Can you work these out from the model? Positions are in its coordinate system, mm. Face numbers are marked on the shaded views. A direction names the side the tool comes from. Round coordinates to 2 decimals unless told otherwise and drop trailing zeros. Order: outer loops, then holes, each group sorted by start corner. A loop starts at its lowest first (then second) coordinate and runs counter-clockwise, first axis right, second up. Notation, with made-up numbers: (89, -10) -> (143, -10) arc R18 cw to (143, 25) -> close; hole circle Ø2 at (58.25, 33). An arc over 180 degrees is marked (long way). One line per item, written item: value.
```python
from build123d import *

# Parameters (mm, degrees)
F0_W     = 40
F0_H     = 40
F1_DEPTH = 40
F2_W     = 20
F2_H     = 20
F3_DEPTH = 20
F7_DEPTH = 24.4958974278


with BuildPart() as f1:
    # F0 (on Front) → F1 (new body)
    with BuildSketch(Plane.XZ):
        with Locations((20, 20)):
            Rectangle(F0_W, F0_H)
    extrude(amount=F1_DEPTH)

    # F2 (on face) → F3 (cut)
    with BuildSketch(Plane.XZ.offset(40)):
        with Locations((30, 30)):
            Rectangle(F2_W, F2_H)
    extrude(amount=-F3_DEPTH, mode=Mode.SUBTRACT)

    # F6 (on 3pt) → F7 (cut, through all)
    with BuildSketch(Plane(origin=(16.6666666667, -16.6666666667, 33.3333333333), x_dir=(0.9128709292, 0.1825741858, -0.3651483717), z_dir=(-0.4082482905, 0.4082482905, -0.8164965809))):
        Polygon((3.6514837167, 26.83281573), (25.5603860169, 8.94427191), (25.5603860169, 31.304951685), align=None)
    extrude(amount=-F7_DEPTH, mode=Mode.SUBTRACT)


solid = f1.part
```
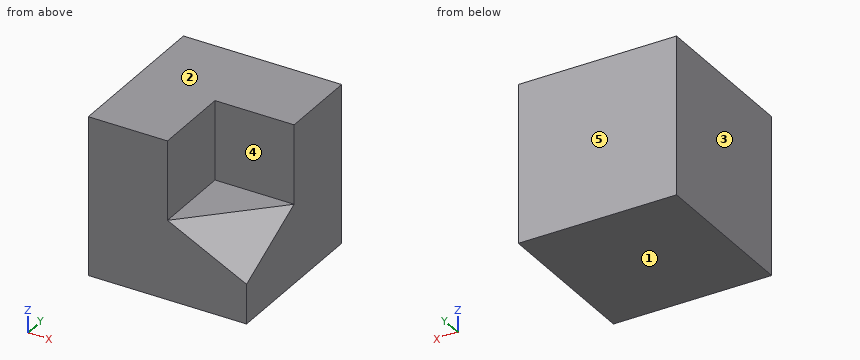
Q1. I want a section at B-B on x = 27. List the corners of the cut face in (y, z) for me.
Answers below:
outline: (-40, 0) -> (0, 0) -> (0, 40) -> (-20, 40) -> (-20, 20) -> (-33, 20) -> (-40, 16.5) -> close
Q2. Will these pins go through, and if not, where does the flat tip stop? pin 1 Ø12 at (y, z) = (-35, 20.5) entering from +X; pin 2 Ø16 at (y, z) = (-31.5, 33.5) entering from +X; pin 3 Ø6 at (x, y) = (27, -26) entering from +Z.
Answers below:
pin 1: x = 37.42
pin 2: x = 20
pin 3: z = 20
Q3. I want a section at D-D on z = 14. List the corners of the cut face in (x, y) for me, plus the area to 3 significant figures.
Answers below:
outline: (0, -40) -> (32, -40) -> (40, -32) -> (40, 0) -> (0, 0) -> close
area: 1,570 mm^2
Q4. I want a section at C-C on z = 19. List the corners of the cut face in (x, y) for me, plus the area to 3 significant figures.
Answers below:
outline: (0, -40) -> (22, -40) -> (40, -22) -> (40, 0) -> (0, 0) -> close
area: 1,440 mm^2
Q5. I want a section at A-A on y = -29. List the corners of the cut face in (x, z) for me, plus the area to 3 significant figures.
Answers below:
outline: (0, 0) -> (40, 0) -> (40, 15.5) -> (31, 20) -> (20, 20) -> (20, 40) -> (0, 40) -> close
area: 1,180 mm^2
Q6. We'd pull the mould along Z, two halves only. Please class the marked faces 1, 2 and 3: released by +Z, released by -Z, zero draft, split by the parting line, or undercut.
Answers below:
face 1: released by -Z
face 2: released by +Z
face 3: zero draft
Q7. Please list where these lines run through material, in increasing order: line 1 along Z through (x, y) = (21, -35); line 2 along Y through (x, z) = (21.5, 37.5).
Answers below:
line 1: 0 to 20
line 2: -20 to 0
Q8. On a 3-axis mill with a long thin cutter (end or side, diameter ignored), from which of +Z, -Z, +X, -X, +Y, -Y can I reach the whole of each face in a straight line? I mean the marked faces 4 and 5. Say none if no direction works.
Answers below:
face 4: +Z, +X, -Y
face 5: +Z, -Z, +X, -X, +Y
